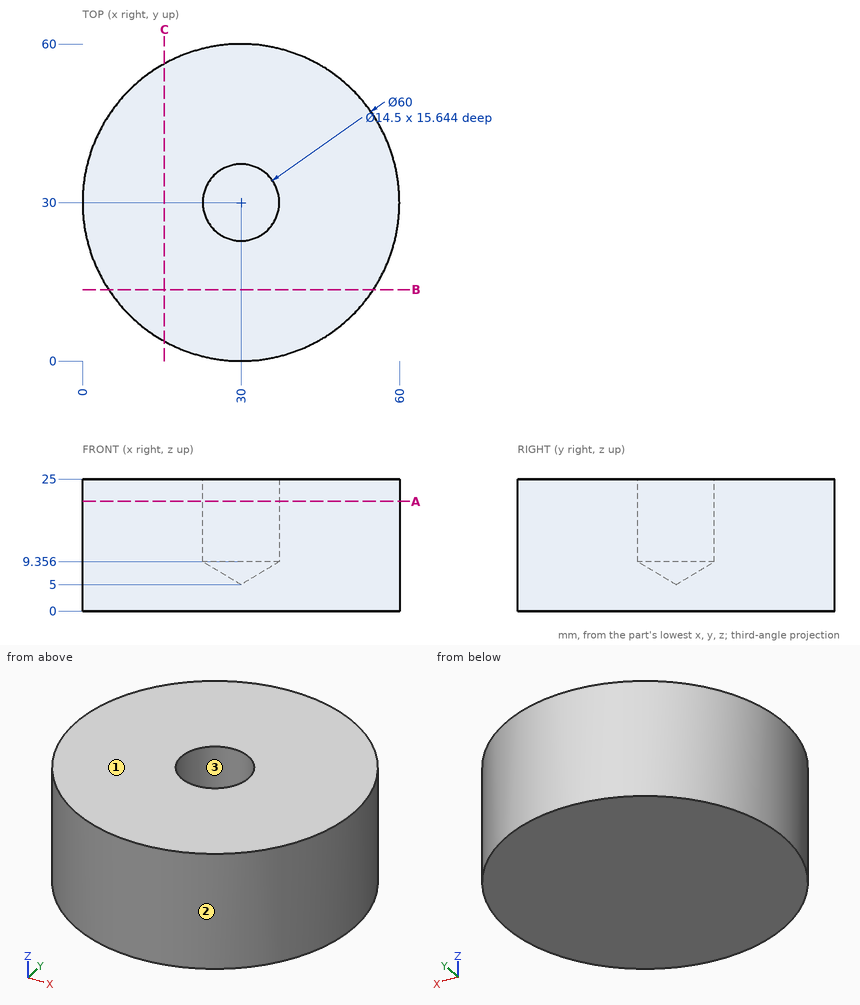
Check sheet for the drawn part. Datum: minimum x, y, z corner. Units: mm. Round coordinates to 2 decimals unless told otherwise and drop trailing zeros. Loops run counter-clockwise (first coordinate to the right, second up) from the corner with the lowest first, then second, coordinate; pieces in that order, holes last. Notation, with made-up numbers: (13, 82.5) - (72, 82.5) arc R11 ccw to (72, 87.5) - close; hole circle Ø6 at (-39.75, 12). An arc over 180 degrees is marked (long way). Write item = value, one per line. Start each with the question number.
1. Section check A-A on z = 20.75. Enter the section's corners in (x, y), then the cut area to 3 significant figures.
2. Section check B-B on y = 13.5. Enter the section's corners in (x, z) (1 decimal), then the cut area to 3 significant figures.
3. Mould release check, pull along Y, two halves, no side actions. Record for the marked faces 1, 2 and 3: released by +Y, released by -Y, zero draft, split by the parting line, or undercut.
4. Depth check by flat-ended pin: pin 1 (1.5 mm diameter, centred on x = 15.5, z = 6, fed in from +Y); pin 2 (10 mm diameter, centred on x = 37.5, z = 17, fed in from +Y); pin 3 (2 mm diameter, centred on x = 48.5, z = 22, fed in from +Y); pin 4 (4 mm diameter, centred on x = 46, y = 39, fed in from -Z). Enter the tip coordinate at first touch or a pass-through.
5. Section check C-C on x = 15.5. Enter the section's corners in (y, z), then the cut area to 3 significant figures.
6. Thickness scan on line 1 (Y direction, x = 30, z = 12.5); line 2 (X direction, y = 25.5, z = 18.5) (1 decimal); line 3 (Y direction, x = 27, z = 17). Record the ranges inside material, lowest first.
Working result:
q1.outline = circle Ø60 at (30, 30); hole circle Ø14.5 at (30, 30)
q1.area = 2,660 mm^2
q2.outline = (4.9, 0) - (55.1, 0) - (55.1, 25) - (4.9, 25) - close
q2.area = 1,250 mm^2
q3.face_1 = zero draft
q3.face_2 = split by the parting line
q3.face_3 = undercut
q4.pin_1 = 56.66
q4.pin_2 = 59.9
q4.pin_3 = 54.37
q4.pin_4 = 0
q5.outline = (3.74, 0) - (56.26, 0) - (56.26, 25) - (3.74, 25) - close
q5.area = 1,310 mm^2
q6.line_1 = 0 to 22.75, 37.25 to 60
q6.line_2 = 0.3 to 24.3, 35.7 to 59.7
q6.line_3 = 0.15 to 23.4, 36.6 to 59.85
